Design review of the part built by this model. Coordinates are the model's own, in mm. Coordinates: 2 decimals unless noted, no trailing zeros. Loops run counter-clockwise (first coordinate to the right, second up) from the corner with the lowest first, then second, coordinate; pieces in that order, holes last. Notation, with made-up numbers: M -17.5,15 L 10.5,15 A21 cw 10.5,43 Z; hole C 64.25,41.5 d2. An arc over 180 degrees is marked long. One line per item, written item: value.
Autodesk Fusion 360 part; units mm, degrees
sketch "Sketch1" plane through (0, 0, 0) normal (0, 0, 1) x (1, 0, 0)
sphere "SpherePrimitive1" add diameter 100 placed x (1, 0, 0) y (0, 1, 0) z (0, 0, 1) at (0, 0, 0)
sketch "Sketch2" plane through (0, 0, 0) normal (1, 0, 0) x (0, 1, 0)
  line L0 (75, 50) -> (-75, 50)
  line L1 (-75, 50) -> (-75, -50)
  line L2 (-75, -50) -> (75, -50)
  line L3 (75, -50) -> (75, 50)
extrude "Extrude1" cut sketch "Sketch2" along normal blind 50
shell "Shell1" thickness 10 removed faces 1 at (0, -9.8252, -7.4174)
(1) We need section D-D on x = -34.5. State the section outline as (y, z) points.
Reply:
outline: C 0,0 d72.38
(2) We need section C-C on y = 36.5. State the section outline as (x, z) points, then the cut area to 3 significant figures.
Reply:
outline: M 0,-34.17 L 0,34.17 A34.17 ccw Z
area: 1,830 mm2
(3) We need section B-B on x = -26. State the section outline as (y, z) points, then the cut area to 3 significant figures.
Reply:
outline: C 0,0 d85.42
area: 5,730 mm2
(4) Insertion check: pin 1 (5 mm diameter, centred on y = 23, z = 7.5, fed in from -X); pin 2 (3 mm diameter, centred on x = -33.5, z = 24.5, fed in from -Y); pin 3 (10 mm diameter, centred on x = -11, y = -16, fed in from -Z). Each pin has a flat end and moves straight along its axis. Give the tip position at first contact, or say it passes through.
Reply:
pin 1: stops at x = -45.05
pin 2: stops at y = -30
pin 3: stops at z = -47.88
(5) We need section A-A on z = 30. State the section outline as (x, y) points, then the cut area to 3 significant figures.
Reply:
outline: M 0,-40 L 0,40 A40 ccw Z
area: 2,510 mm2
(6) To check wall thickness, follow line 1 along Y through (x, z) = (-7, -34.5); line 2 along Z through (x, y) = (-19, -11.5); line 3 along Y through (x, z) = (-19, -35.5). State the ranges of each line that lie inside material, in increasing order. Write a range as [from, to].
Reply:
line 1: y = [-35.51, 35.51]
line 2: z = [-44.8, 44.8]
line 3: y = [-29.64, 29.64]
